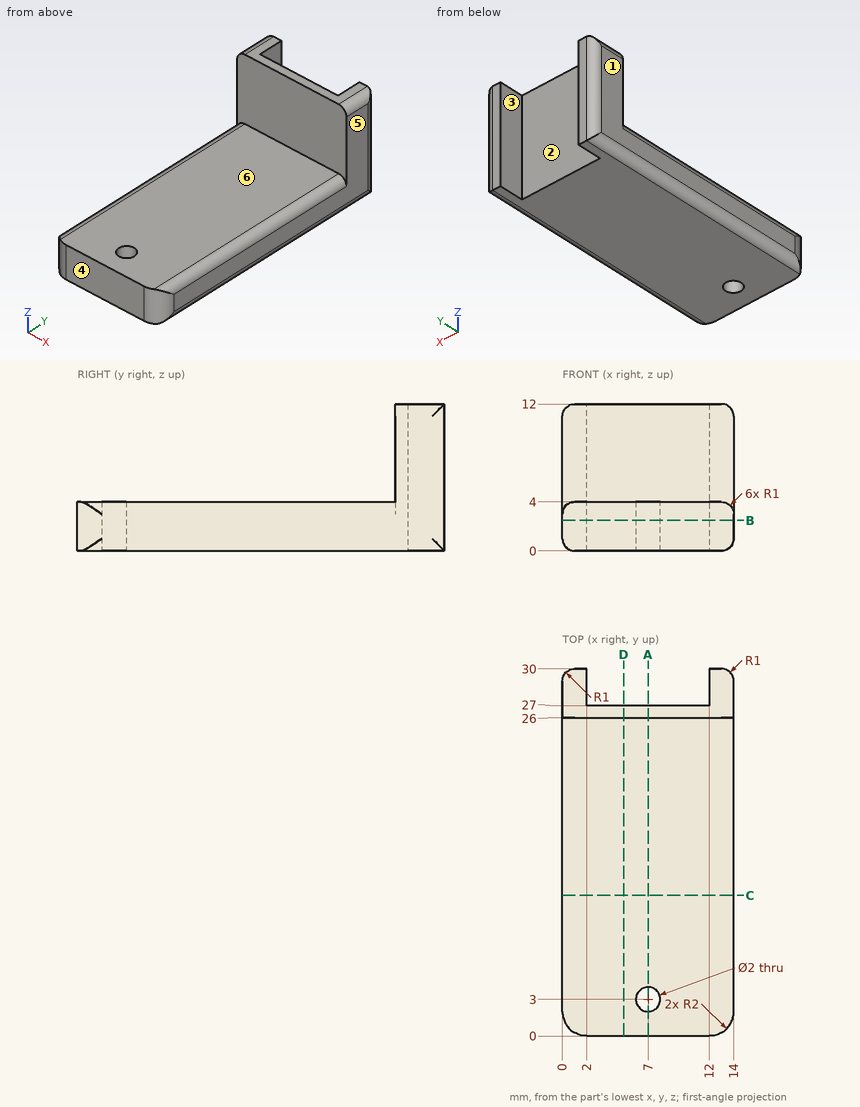
Here's the drawing with two shaded views (mm, measured from the low corner). I have some questions. A direction names the side the tool comes from. Round coordinates to 2 decimals unless told otherwise and drop trailing zeros. Loops run counter-clockwise (first coordinate to the right, second up) from the corner with the lowest first, then second, coordinate; pieces in that order, holes last.
Item 1: Suppose I cut it at C-C, the plane y = 11.5. Write out the boundary of the cut face in (x, z).
Item 2: Will these pins go through, and if not, where does the flat tip stop? pin 1 Ø2.5 at (x, z) = (5.5, 7.5) entering from -Y; pin 2 Ø3 at (x, y) = (4, 7) entering from +Z; pin 3 Ø1 at (y, z) = (14.5, 4) entering from +X.
Item 3: Suppose I cut it at D-D, the plane x = 5. Write out the boundary of the cut face in (y, z).
Item 4: Suppose I cut it at A-A, the plane x = 7. Write out the boundary of the cut face in (y, z), then the cut area to 3 significant figures.
Item 5: If we mould it in two halves opening along X, with no side actions, what happens to the marked faces 1, 2, 3 and 4? For each: +X half, -X half, draft (parallel to the pull), parting line (faces both ways), or undercut.
Item 6: Which directions (+Z, -Z, +X, -X, +Y, -Y) give clear straight access to the entire face, cutting with the end or side of a thin tool? Please do the marked faces 5 and 6.
Item 7: Please list where these lines run through material, in increasing order: L1, parallel to Y at x = 7, z = 2.5; L2, parallel to Y at x = 8.75, z = 6.5; L3, parallel to Y at x = 1.25, z = 9.5.
Item 8: Suppose I cut it at B-B, the plane z = 2.5. Write out the boundary of the cut face in (x, y).
Reported:
1. outline: (0, 1) arc R1 ccw to (1, 0) - (13, 0) arc R1 ccw to (14, 1) - (14, 3) arc R1 ccw to (13, 4) - (1, 4) arc R1 ccw to (0, 3) - close
2. pin 1: stops at y = 26
2. pin 2: stops at z = 4
2. pin 3: stops at x = 13.87
3. outline: (0, 0) - (27, 0) - (27, 12) - (26, 12) - (26, 4) - (0, 4) - close
4. outline: (0, 0) - (2, 0) - (2, 4) - (0, 4) - close; (4, 0) - (27, 0) - (27, 12) - (26, 12) - (26, 4) - (4, 4) - close
4. area: 108 mm2
5. face 1: -X half
5. face 2: undercut
5. face 3: undercut
5. face 4: draft
6. face 5: +Z, -Z, +X, +Y, -Y
6. face 6: +Z, +X, -X, -Y
7. L1: y = 0 to 2, 4 to 27
7. L2: y = 26 to 27
7. L3: y = 26 to 30
8. outline: (0, 2) arc R2 ccw to (2, 0) - (12, 0) arc R2 ccw to (14, 2) - (14, 29) arc R1 ccw to (13, 30) - (12, 30) - (12, 27) - (2, 27) - (2, 30) - (1, 30) arc R1 ccw to (0, 29) - close; hole circle Ø2 at (7, 3)
